Verification items for this drawing (mm, ordinates from the low corner). A direction names the side the tool comes from. Round coordinates to 2 decimals unless told otherwise and drop trailing zeros. Loops run counter-clockwise (first coordinate to the right, second up) from the corner with the lowest first, then second, coordinate; pieces in that order, holes last. Notation, with made-up numbers: M -17,68 L 21,68 A33 ccw 21,99 Z; hole C 37.25,57.25 d3. An arc over 180 degrees is marked long. One line per item, written item: value.
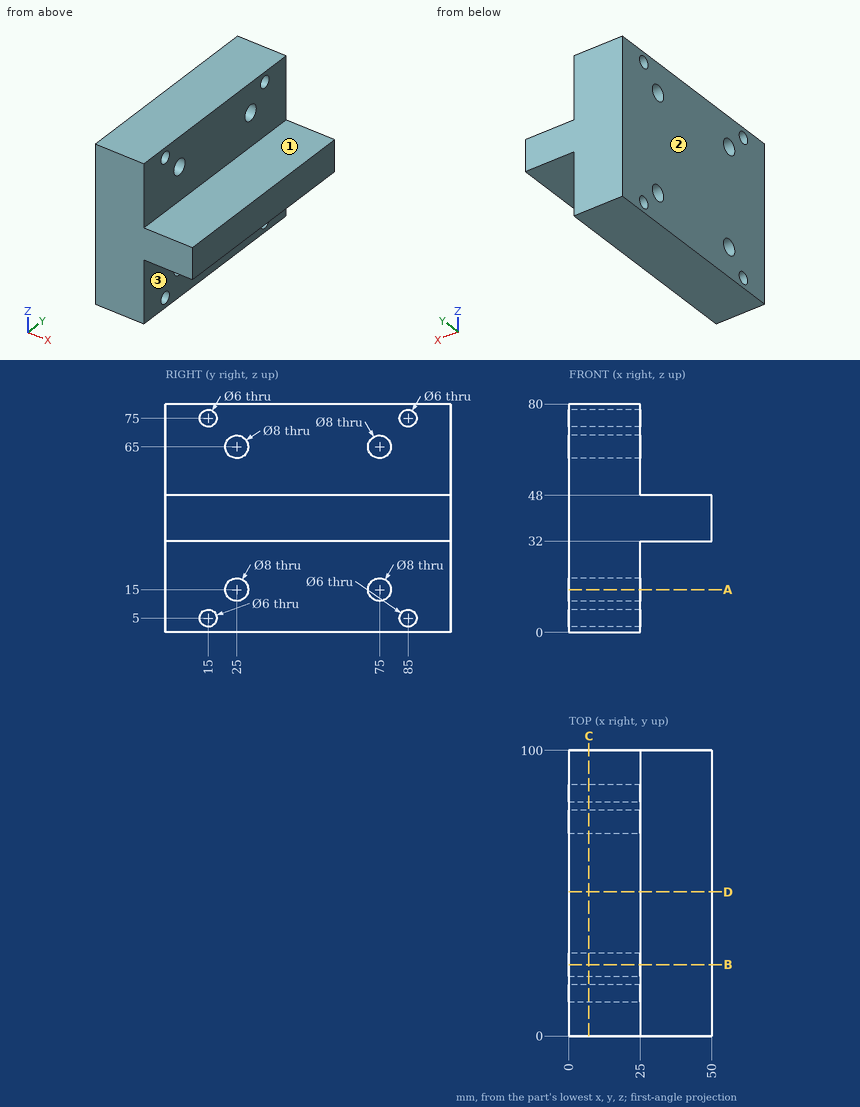
(1) Tool access check on the marked faces 1, 2 and 3. Record the directions out of +Z, -Z, +X, -X, +Y, -Y that give a thin tool (end or side, any length) a straight path to the whole face; none if there is none.
Completed:
face 1: +Z, +X, +Y, -Y
face 2: +Z, -Z, -X, +Y, -Y
face 3: -Z, +X, +Y, -Y
(2) Sectioned sample at A-A on z = 15. Enter the section's corners in (x, y).
Completed:
outline: M 0,0 L 25,0 L 25,21 L 0,21 Z; M 0,29 L 25,29 L 25,71 L 0,71 Z; M 0,79 L 25,79 L 25,100 L 0,100 Z
(3) Sectioned sample at D-D on y = 50.5. Enter the section's corners in (x, z), and give its area (3 significant figures).
Completed:
outline: M 0,0 L 25,0 L 25,32 L 50,32 L 50,48 L 25,48 L 25,80 L 0,80 Z
area: 2,400 mm^2
(4) Sectioned sample at C-C on x = 7. Count the separate pieces of the cut face and the enclosed holes in it, and give its area (3 significant figures).
Completed:
separate pieces: 1
enclosed holes: 8
area: 7,690 mm^2
(5) Sectioned sample at B-B on y = 25. Enter the section's corners in (x, z), and give its area (3 significant figures).
Completed:
outline: M 0,0 L 25,0 L 25,11 L 0,11 Z; M 0,19 L 25,19 L 25,32 L 50,32 L 50,48 L 25,48 L 25,61 L 0,61 Z; M 0,69 L 25,69 L 25,80 L 0,80 Z
area: 2,000 mm^2
(6) Depth check by flat-ended pin: pin 1 Ø3 at (x, z) = (18.5, 17.5) entering from -Y; pin 2 Ø5 at (y, z) = (24.5, 21.5) entering from +X; pin 3 Ø3.5 at (y, z) = (85, 5) entering from -X; pin 4 Ø5 at (x, y) = (42.5, 12) entering from -Z. Enter the tip coordinate at first touch or a pass-through.
Completed:
pin 1: stops at y = 0
pin 2: stops at x = 25
pin 3: passes through
pin 4: stops at z = 32
(7) Thickness scan on L1, parallel to Z at x = 6, y = 75; L2, parallel to Z at x = 10, y = 85; L3, parallel to Y at x = 24, z = 64. Record the ranges inside material, lowest first. Write a range as from..to.
Completed:
L1: z = 0..11, 19..61, 69..80
L2: z = 0..2, 8..72, 78..80
L3: y = 0..21.13, 28.87..71.13, 78.87..100
